Geometry: final body of the model. Coordinates: model frame, mm. Coordinates: 2 decimals unless noted, no trailing zeros. Write each loop counter-clockwise with the first axis right and the second up, starting at its lowest first coordinate (ties: lowest second). Pieces come first, ordered by that corner, then holes. Notation, with made-up numbers: (79, 21) - (110, 21) arc R25 cw to (110, 38) - close; hole circle Ø8 at (18, 27.25). An arc over 180 degrees is marked (long way). Answer as a JSON object with one key per item and string values. Group by question number.
Item 1: Mould query, pull axis Y, two halves, no side actions, for faces 1 (the cylindrical face through (-20.3, 190.42, 1.48)), 2 (the flat face through (-6, 184, 3)), 3 (the cylindrical face through (14.4, 163.07, 1.52)). Classes: pulls with the +Y half, pulls with the -Y half, needs draft (parallel to the pull), parting line crosses it, or undercut.
Item 2: First-contact query: pin 1 Ø2.5 at (x, y) = (7.5, 180) entering from +Z. Flat tip, straight axial feed; report the tip coordinate or a pass-through.
Item 3: Section D-D on x = -21. Return loops of the section in (y, z).
Item 4: Section B-B on y = 171. Return loops of the section in (x, z), and give its area (3 significant figures).
Item 5: Line query: line 1 along Y through (x, z) = (7.5, 0.85); line 2 along X through (y, z) = (189, 1.9); line 3 along X through (y, z) = (190, 0.9). Output: solid intervals per line, ascending. Write a range as from..to.
Item 6: Section A-A on x = 7.5. Return loops of the section in (y, z).
Item 7: Section C-C on z = 1. Return loops of the section in (x, y), and give its area (3 significant figures).
Autodesk Inventor part; units mm, degrees
ref_plane "作業平面1" through (0, 0, 0) normal (0, 0, 1) x (1, 0, 0)
ref_plane "YZ Plane" through (0, 0, 0) normal (1, 0, 0) x (0, 1, 0)
ref_plane "XZ Plane" through (0, 0, 0) normal (0, 1, 0) x (-1, 0, 0)
ref_plane "作業平面1" through (0, 0, 0) normal (0, 0, 1) x (1, 0, 0)
sketch "スケッチ1" plane through (0, 0, 0) normal (0, 0, 1) x (1, 0, 0)
  circle A0 centre (7.5, 170) radius 1.6
  circle A1 centre (7.5, 180) radius 1.6
  circle A2 centre (7.5, 190) radius 1.6
  circle A3 centre (-11.0383, 189) radius 1.6
  circle A4 centre (-21.0383, 189) radius 1.6
  circle A5 centre (-31.0383, 189) radius 1.6
  line L0 (15, 162.5) -> (0, 162.5)
  line L1 (0, 162.5) -> (-38.5383, 181.5)
  line L2 (-38.5383, 181.5) -> (-38.5383, 196.5)
  line L3 (-38.5383, 196.5) -> (15, 196.5)
  line L4 (15, 196.5) -> (15, 162.5)
  point P0 (0, 0)
  dimension "d0" = 7.5
  dimension "d1" = 7.5
  dimension "d2" = 7.5
  dimension "d3" = 7.5
  dimension "d4" = 7.5
  dimension "d5" = 7.5
extrude "押し出し1" add sketch "スケッチ1" along normal blind 3
fillet "フィレット1" radius 2 5 edges at (15, 162.5, 1.5) (15, 196.5, 1.5) (-38.5383, 196.5, 1.5) (-38.5383, 181.5, 1.5) (0, 162.5, 1.5)
properties part number "オムニ_koteigu" material "アルミニウム 6061"
Checks:
{
 "1": {"face 1": "undercut", "face 2": "needs draft", "face 3": "pulls with the -Y half"},
 "2": {"pin 1": "through"},
 "3": {"outline": "(172.85, 0) - (187.4, 0) - (187.4, 3) - (172.85, 3) - close; (190.6, 0) - (196.5, 0) - (196.5, 3) - (190.6, 3) - close"},
 "4": {"outline": "(-17.24, 0) - (6.25, 0) - (6.25, 3) - (-17.24, 3) - close; (8.75, 0) - (15, 0) - (15, 3) - (8.75, 3) - close", "area": "89.2 mm^2"},
 "5": {"line 1": "162.5..168.4, 171.6..178.4, 181.6..188.4, 191.6..196.5", "line 2": "-38.54..-32.64, -29.44..-22.64, -19.44..-12.64, -9.44..6.25, 8.75..15", "line 3": "-38.54..-32.29, -29.79..-22.29, -19.79..-12.29, -9.79..5.9, 9.1..15"},
 "6": {"outline": "(162.5, 0) - (168.4, 0) - (168.4, 3) - (162.5, 3) - close; (171.6, 0) - (178.4, 0) - (178.4, 3) - (171.6, 3) - close; (181.6, 0) - (188.4, 0) - (188.4, 3) - (181.6, 3) - close; (191.6, 0) - (196.5, 0) - (196.5, 3) - (191.6, 3) - close"},
 "7": {"outline": "(-38.54, 182.74) arc R2 ccw to (-37.42, 180.95) - (-0.42, 162.71) arc R2 ccw to (0.47, 162.5) - (13, 162.5) arc R2 ccw to (15, 164.5) - (15, 194.5) arc R2 ccw to (13, 196.5) - (-36.54, 196.5) arc R2 ccw to (-38.54, 194.5) - close; hole circle Ø3.2 at (-31.04, 189); hole circle Ø3.2 at (-21.04, 189); hole circle Ø3.2 at (-11.04, 189); hole circle Ø3.2 at (7.5, 170); hole circle Ø3.2 at (7.5, 180); hole circle Ø3.2 at (7.5, 190)", "area": "1,400 mm^2"}
}
